from build123d import *

# Parameters (mm, degrees)
SKETCH_1_W                 = 20
SKETCH_1_H                 = 32.5
SKETCH_1_R                 = 1.3
EXTRUDE_1_DEPTH            = 1.5
SKETCH_2_R                 = 9.8
EXTRUDE_2_DEPTH            = 5.8
FILLET_1_R                 = 1
SKETCH_4_W                 = 6.7
SKETCH_4_H                 = 6.7
EXTRUDE_3_DEPTH            = 4.8
SKETCH_5_R                 = 0.5
EXTRUDE_4_DEPTH            = 4.6
SKETCH_6_W                 = 2.5
SKETCH_6_H                 = 2.5
EXTRUDE_5_DEPTH            = 3.7
EXTRUDE_6_DEPTH            = 0.3
PATTERN_LINEAR_1_COUNT     = 3
PATTERN_LINEAR_1_PITCH     = 2.5
PATTERN_LINEAR_1_COL_COUNT = 2
PATTERN_LINEAR_1_COL_PITCH = 2.5


with BuildPart() as part:
    # 草图1 → 凸台-拉伸1 (new body)
    with BuildSketch(Plane(origin=(0, 0, 0), x_dir=(1, 0, 0), z_dir=(0, 1, 0))):
        Rectangle(SKETCH_1_W, SKETCH_1_H)
        with Locations((7.6, 13.5)):
            Circle(SKETCH_1_R, mode=Mode.SUBTRACT)
        with Locations((-7.6, 13.5)):
            Circle(SKETCH_1_R, mode=Mode.SUBTRACT)
        with Locations((-7.6, -13.5)):
            Circle(SKETCH_1_R, mode=Mode.SUBTRACT)
        with Locations((7.6, -13.5)):
            Circle(SKETCH_1_R, mode=Mode.SUBTRACT)
    extrude(amount=EXTRUDE_1_DEPTH)

    # 草图2 → 凸台-拉伸2 (add)
    with BuildSketch(Plane(origin=(0, 1.5, 0), x_dir=(1, 0, 0), z_dir=(0, 1, 0))):
        with Locations((0, 3.65)):
            Circle(SKETCH_2_R)
    extrude(amount=EXTRUDE_2_DEPTH)

    # 草图3 → 旋转1 (revolve)
    with BuildSketch(Plane(origin=(0, 0, 0), x_dir=(0, 0, -1), z_dir=(1, 0, 0))):
        Polygon((3.65, 7.163786099), (11.65, 7.163786099), (9.65, 16.363786099), (3.65, 16.363786099), align=None)
    revolve(axis=Axis((0, 2.048350332, -3.65), (0, 1, 0)))

    # 圆角1
    fillet_1_edges = [part.edges().sort_by_distance(p)[0] for p in [
        (0, 16.363786099, 2.35),
    ]]
    fillet(fillet_1_edges, radius=FILLET_1_R)

    # 草图4 → 凸台-拉伸3 (add)
    with BuildSketch(Plane.XZ):
        with Locations((-6.45, 8.1)):
            Rectangle(SKETCH_4_W, SKETCH_4_H)
    extrude(amount=EXTRUDE_3_DEPTH)

    # 草图5 → 凸台-拉伸4 (add)
    with BuildSketch(Plane.XZ):
        with Locations((4.75, -3.65)):
            Circle(SKETCH_5_R)
        with Locations((3.358757211, -7.008757211)):
            Circle(SKETCH_5_R)
        with Locations((-3.358757211, -7.008757211)):
            Circle(SKETCH_5_R)
        with Locations((-4.75, -3.65)):
            Circle(SKETCH_5_R)
        with Locations((-3.358757211, -0.291242789)):
            Circle(SKETCH_5_R)
        with Locations((3.358757211, -0.291242789)):
            Circle(SKETCH_5_R)
    extrude(amount=EXTRUDE_4_DEPTH)

    # 草图6 → 凸台-拉伸5 (add)
    with BuildSketch(Plane.XZ):
        with Locations((1.25, 14.6)):
            Rectangle(SKETCH_6_W, SKETCH_6_H)
    extrude_5 = extrude(amount=EXTRUDE_5_DEPTH)

    # 草图7 → 凸台-拉伸6 (add, symmetric)
    with BuildSketch(Plane(origin=(1.25, 0, 0), x_dir=(0, 0, -1), z_dir=(1, 0, 0))):
        with BuildLine():
            Line((-14.3, 1.9), (-14.9, 1.9))
            Line((-14.9, 1.9), (-14.9, -4.1))
            ThreePointArc((-14.9, -4.1), (-15.017157288, -4.382842712), (-15.3, -4.5))
            Line((-15.3, -4.5), (-22.1, -4.5))
            Line((-22.1, -4.5), (-22.1, -5.1))
            Line((-22.1, -5.1), (-15.3, -5.1))
            ThreePointArc((-15.3, -5.1), (-14.592893219, -4.807106781), (-14.3, -4.1))
            Line((-14.3, -4.1), (-14.3, 1.9))
        make_face()
    extrude_6 = extrude(amount=EXTRUDE_6_DEPTH, both=True)

    # 阵列(线性)1: 凸台-拉伸5, 凸台-拉伸6 ×3
    with Locations(*[(-i * PATTERN_LINEAR_1_PITCH, 0, 0) for i in range(1, PATTERN_LINEAR_1_COUNT)]):
        add(extrude_5)
        add(extrude_6)

    # 阵列(线性)1 col: 凸台-拉伸5, 凸台-拉伸6 ×2
    with Locations(*[(i * PATTERN_LINEAR_1_COL_PITCH, 0, 0) for i in range(1, PATTERN_LINEAR_1_COL_COUNT)]):
        add(extrude_5)
        add(extrude_6)


solid = part.part
The listing builds one solid part. Answer for the finished solid, in the listing's coordinates (mm). A direction names the side the tool comes from. Round coordinates to 2 decimals unless told otherwise and drop trailing zeros. Order: outer loops, then holes, each group sorted by start corner. A loop starts at its lowest first (then second) coordinate and runs counter-clockwise, first axis right, second up. Notation, with made-up numbers: (-9, 82.5) -> (35, 82.5) arc R16 ccw to (35, 100.5) -> close; hole circle Ø2 at (-33.75, -6.75). An arc over 180 degrees is marked (long way). One line per item, written item: value.
Item 1: Find section C-C, the plane x = 0. Give the vertices of the cut face in (y, z).
Taken from the geometry:
outline: (-3.7, 13.35) -> (0, 13.35) -> (0, -16.25) -> (1.5, -16.25) -> (1.5, -13.45) -> (7.3, -13.45) -> (7.3, -11.62) -> (15.58, -9.82) arc R1 ccw to (16.36, -8.84) -> (16.36, 1.54) arc R1 ccw to (15.58, 2.52) -> (7.3, 4.32) -> (7.3, 6.15) -> (1.5, 6.15) -> (1.5, 16.25) -> (0, 16.25) -> (0, 15.85) -> (-3.7, 15.85) -> close
Item 2: For a pull along Z with two mould halves and no side action, classify faces 5 (the flat face through (-10, 1, 0)), 6 (the flat face through (0, 1, 16.25)), 7 (the flat face through (-3.1, -2, 8)) as released by +Z, released by -Z, zero draft, split by the parting line, or undercut.
Taken from the geometry:
face 5: zero draft
face 6: released by +Z
face 7: undercut
Item 3: Given P1, Ø6, axis at y = 10, z = 8.5, coming from the +X side; P2, Ø1.5, axis at y = -4.5, z = 20, coming from the +X side; P3, Ø6, axis at x = -5, y = -1, coming from the +Z side; P4, Ø1, axis at x = 1, z = 9, coming from the -Y side, each flat-ended and moving along its own axis, determine where each tip first touches the part or whether it passes through.
Taken from the geometry:
P1: passes through
P2: stops at x = 4.05
P3: stops at z = 16.25
P4: stops at y = 0
Item 4: Find section A-A, the plane z = 19. Give the vertices of the cut face in (x, y).
Taken from the geometry:
outline: (-4.05, -5.1) -> (-3.45, -5.1) -> (-3.45, -4.5) -> (-4.05, -4.5) -> close; (-1.55, -5.1) -> (-0.95, -5.1) -> (-0.95, -4.5) -> (-1.55, -4.5) -> close; (0.95, -5.1) -> (1.55, -5.1) -> (1.55, -4.5) -> (0.95, -4.5) -> close; (3.45, -5.1) -> (4.05, -5.1) -> (4.05, -4.5) -> (3.45, -4.5) -> close
Item 5: Find section D-D, the plane z = 8. Give the vertices of the cut face in (x, y), then the cut area to 3 significant figures.
Taken from the geometry:
outline: (-10, 0) -> (-9.8, 0) -> (-9.8, -4.8) -> (-3.1, -4.8) -> (-3.1, 0) -> (10, 0) -> (10, 1.5) -> (-10, 1.5) -> close
area: 62.2 mm2
Item 6: Find section B-B, the plane y = -1. Give the vertices of the cut face in (x, z), then the cut area to 3 significant figures.
Taken from the geometry:
outline: (-9.8, 4.75) -> (-3.1, 4.75) -> (-3.1, 11.45) -> (-9.8, 11.45) -> close; circle Ø1 at (-4.75, -3.65); (-5, 13.35) -> (5, 13.35) -> (5, 15.85) -> (-5, 15.85) -> close; circle Ø1 at (-3.36, -7.01); circle Ø1 at (-3.36, -0.29); circle Ø1 at (3.36, -7.01); circle Ø1 at (3.36, -0.29); circle Ø1 at (4.75, -3.65)
area: 74.6 mm2
Item 7: Straight lines are drawn through the part: L1, parallel to Z at x = 7.6, y = 0.9; L2, parallel to X at y = 0.5, z = -13.5; L3, parallel to Z at x = -4, y = -3.25. For each, find the intervals that lie inside material, in ascending order.
Taken from the geometry:
L1: z = -16.25 to -14.8, -12.2 to 12.2, 14.8 to 16.25
L2: x = -10 to -8.9, -6.3 to 6.3, 8.9 to 10
L3: z = 4.75 to 11.45, 13.35 to 15.85
Item 8: For faces 1 (the flat face through (-6, -2, 4.75)), 2 (the cylindrical face through (3.82, -2.27, -0.48)), 3 (the flat face through (-5, -2, 15)), 4 (the flat face through (-0.95, -4.7, 18.3)), determine the directions among +Z, -Z, +X, -X, +Y, -Y from which every point of the face is accessible in a straight line to the end or side of a thin tool.
Taken from the geometry:
face 1: +X, -X, -Y
face 2: -Y
face 3: +Z, -X, -Y
face 4: +Z, -Z, -Y
